Autodesk Inventor part; units mm, degrees
ref_plane "YZ Plane" through (0, 0, 0) normal (1, 0, 0) x (0, 1, 0)
ref_plane "XZ Plane" through (0, 0, 0) normal (0, 1, 0) x (-1, 0, 0)
ref_plane "XY Plane" through (0, 0, 0) normal (0, 0, 1) x (1, 0, 0)
sketch "Sketch3" plane through (0, 0, 0) normal (0, 1, 0) x (-1, 0, 0)
  circle A0 centre (0, 0) radius 6.5
  circle A1 centre (0, 0) radius 5
  dimension "d4" = 13
  dimension "d6" = 10
extrude "Extrusion2" add sketch "Sketch3" along normal blind 80
fillet "Fillet1" radius 0.3 2 edges at (6.5, 0, 0) (5, 0, 0)
fillet "Fillet2" radius 0.3 1 edges at (6.5, 80, 0)
fillet "Fillet3" radius 0.3 1 edges at (5, 80, 0)
properties part number "tube_long" material "Glass"
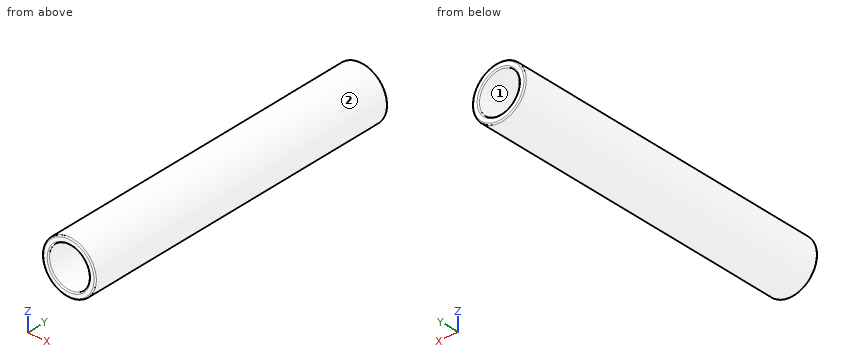
Input: part model. Units: mm. Frame: model coordinates. Face numbers are marked on the shaded views. Give positions to 0.01 mm unless a question says otherwise; leave off trailing zeros. Loops run counter-clockwise (first coordinate to the right, second up) from the corner with the lowest first, then second, coordinate; pieces in that order, holes last. Notation, with made-up numbers: (86.25, 30.5) -> (120.25, 30.5) arc R24 cw to (120.25, 66.5) -> close; hole circle Ø9 at (16, 53). An arc over 180 degrees is marked (long way). Answer as a JSON object with one key per item and string values. Group by question number.
Item 1: Line query: probe 1 along Z at (x, y) = (0, 51); probe 2 along X at (y, z) = (30.5, 0.25); probe 3 along Z at (x, y) = (4.25, 40). Output: solid intervals per line, ascending.
Item 2: Cut plane B-B, the plane x = 0. Return the cut outline in (y, z).
Item 3: Pull-direction query (X, two-part tool) for the marked faces 1 and 2; classes: released by +X, released by -X, zero draft, split by the parting line, or undercut.
Item 4: Pin query (flat end, axial travel): P1, Ø4, axis at x = 4, y = 40, coming from the -Z side; P2, Ø3, axis at y = 37, z = 5, coming from the -X side; P3, Ø4, axis at y = 69.5, z = 2.5, coming from the -X side; P4, Ø2, axis at x = 3.5, z = 3.5, coming from the +Y side. Return the tip coordinate at first contact, or that it passes through.
Item 5: Cut plane C-C, the plane y = 22.5. Return the cut outline in (x, z), and give its area (3 significant figures).
Item 6: Cut plane A-A, the plane z = 0. Return the cut outline in (x, y).
Checks:
{
 "1": {"probe 1": "z = -6.5 to -5, 5 to 6.5", "probe 2": "x = -6.5 to -4.99, 4.99 to 6.5", "probe 3": "z = -4.92 to -2.63, 2.63 to 4.92"},
 "2": {"outline": "(0, -6.2) arc R0.3 ccw to (0.3, -6.5) -> (79.7, -6.5) arc R0.3 ccw to (80, -6.2) -> (80, -5.3) arc R0.3 ccw to (79.7, -5) -> (0.3, -5) arc R0.3 ccw to (0, -5.3) -> close; (0, 5.3) arc R0.3 ccw to (0.3, 5) -> (79.7, 5) arc R0.3 ccw to (80, 5.3) -> (80, 6.2) arc R0.3 ccw to (79.7, 6.5) -> (0.3, 6.5) arc R0.3 ccw to (0, 6.2) -> close"},
 "3": {"face 1": "undercut", "face 2": "split by the parting line"},
 "4": {"P1": "stops at z = -6.18", "P2": "stops at x = -5.48", "P3": "stops at x = -6.48", "P4": "stops at y = 80"},
 "5": {"outline": "circle Ø13 at (0, 0); hole circle Ø10 at (0, 0)", "area": "54.2 mm²"},
 "6": {"outline": "(-6.5, 0.3) arc R0.3 ccw to (-6.2, 0) -> (-5.3, 0) arc R0.3 ccw to (-5, 0.3) -> (-5, 79.7) arc R0.3 ccw to (-5.3, 80) -> (-6.2, 80) arc R0.3 ccw to (-6.5, 79.7) -> close; (5, 0.3) arc R0.3 ccw to (5.3, 0) -> (6.2, 0) arc R0.3 ccw to (6.5, 0.3) -> (6.5, 79.7) arc R0.3 ccw to (6.2, 80) -> (5.3, 80) arc R0.3 ccw to (5, 79.7) -> close"}
}
